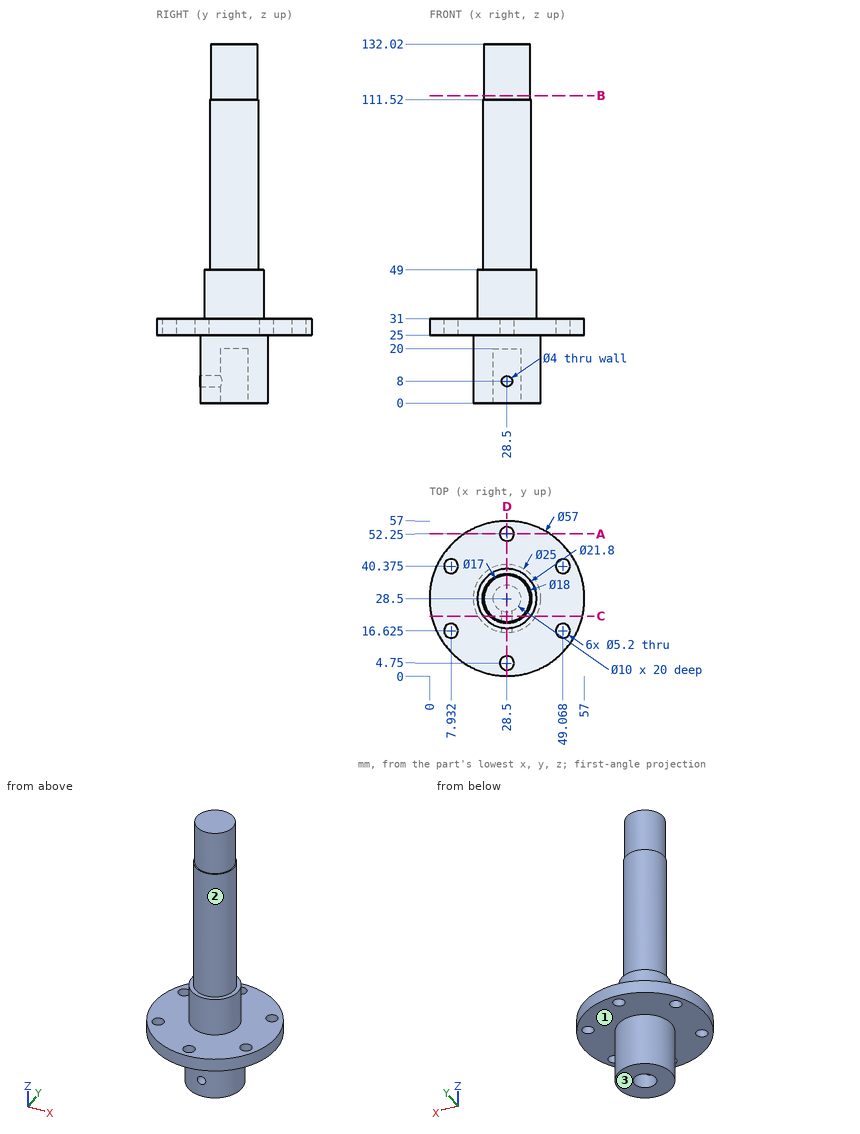
Drawing for the job (mm, zero at the part's lowest x, y, z). A direction names the side the tool comes from. Round coordinates to 2 decimals unless told otherwise and drop trailing zeros. Loops run counter-clockwise (first coordinate to the right, second up) from the corner with the lowest first, then second, coordinate; pieces in that order, holes last. Notation, with made-up numbers: (-33.5, 27) -> (-0.5, 27) arc R21 cw to (-0.5, 51) -> close; hole circle Ø6 at (75, 58.25). An arc over 180 degrees is marked (long way). Use one line per item in the form item = value. Start each with the question number.
Item 1: Band-saw the part on B-B (z = 113). List the corners of the cut face in (x, y).
Item 2: Band-saw the part on D-D (x = 28.5). Give the number of separate pieces and of enclosed holes in the cut face, plus the area to 3 significant figures.
Item 3: Band-saw the part on A-A (y = 52.25). List the corners of the cut face in (x, z).
Item 4: Drill centre lines: line 1 along Y through (x, z) = (28.5, 28.3); line 2 along Y through (x, z) = (28.5, 15.25); line 3 along Z through (x, y) = (3, 20.5). Where is each one in solid material? Low to high.
Item 5: Drop flat-ended pins along their axis: pin 1 Ø5 at (x, y) = (49.5, 43.5) entering from -Z; pin 2 Ø4 at (x, y) = (47.5, 7.5) entering from +Z; pin 3 Ø3 at (y, z) = (28.5, 55.5) entering from -X. Give the stop position or say it passes through.
Item 6: Band-saw the part on C-C (y = 22). List the corners of the cut face in (x, z) (3 decimals), plus the area to 3 significant figures.
Item 7: Tool access for the marked faces 1, 2 and 3: list every direction of +Z, -Z, +X, -X, +Y, -Y with a clear straight run to the whole face (end or side of a thin tool).
Data:
q1.outline = circle Ø17 at (28.5, 28.5)
q2.separate_pieces = 4
q2.enclosed_holes = 0
q2.area = 2,540 mm^2
q3.outline = (12.75, 25) -> (25.9, 25) -> (25.9, 31) -> (12.75, 31) -> close; (31.1, 25) -> (44.25, 25) -> (44.25, 31) -> (31.1, 31) -> close
q4.line_1 = 0 to 2.15, 7.35 to 49.65, 54.85 to 57
q4.line_2 = 16 to 23.5, 33.5 to 41
q4.line_3 = 25 to 31
q5.pin_1 = 25
q5.pin_2 = 31
q5.pin_3 = 19.5
q6.outline = (0.751, 25) -> (17.823, 25) -> (17.823, 0) -> (39.177, 0) -> (39.177, 25) -> (56.249, 25) -> (56.249, 31) -> (37.25, 31) -> (37.25, 49) -> (34.725, 49) -> (34.725, 111.52) -> (33.977, 111.52) -> (33.977, 132.02) -> (23.023, 132.02) -> (23.023, 111.52) -> (22.275, 111.52) -> (22.275, 49) -> (19.75, 49) -> (19.75, 31) -> (0.751, 31) -> close; hole circle Ø4 at (28.5, 8)
q6.area = 2,170 mm^2
q7.face_1 = -Z
q7.face_2 = +Z
q7.face_3 = -Z, +X, -X, +Y, -Y
